Geometry: final body of the model. Coordinates: model frame, mm. A direction names the side the tool comes from. Give positions to 0.01 mm unless a question says otherwise; leave off trailing zeros. Order: outer loops, then holes, each group sorted by start corner. A loop starts at its lowest first (then second) coordinate and runs counter-clockwise, first axis right, second up. Notation, with made-up numbers: (-16, 37.25) - (-1, 37.25) arc R30 ccw to (-1, 70.25) - close; hole circle Ø6 at (38.25, 65). An arc over 180 degrees is marked (long way). Put each result on its own line as item: value. Start each with the question number.
1. Mould query, pull axis Z, two halves, no side actions, for faces 1 (the flat face through (0, -42, 20)), 2 (the flat face through (-5.5, 53, 12)), 3 (the flat face through (10.25, -78, -11)). Classes: pulls with the +Z half, pulls with the -Z half, needs draft (parallel to the pull), parting line crosses it, or undercut.
2. Section D-D on y = 0. Return the cut outline in (x, z), plus the area to 3 significant figures.
3. First-contact query: P1, Ø8.5, axis at x = 7.5, y = 54.5, coming from the -Z side; P2, Ø8, axis at y = 42.5, z = 5, coming from the +X side; P3, Ø9, axis at y = 58, z = 14.5, coming from the +X side; P4, Ø10, axis at x = -32, z = -8, coming from the -Y side. Flat tips, straight axial feed; report the tip coordinate or a pass-through.
4. Set-up query: faces 4 (the flat face through (0, -61.5, -21)), 5 (the flat face through (-17.5, -72, 1)), 6 (the flat face through (17.5, -73, 1)), 7 (the flat face through (7.25, -77, -18)), 8 (the flat face through (5, 49, 0.25)). Return all of +Z, -Z, +X, -X, +Y, -Y with unobstructed straight access to the full face (end or side cutting, diameter ignored); none if empty.
5. Ray query, line 1 along X through (y, z) = (0, 16); line 2 along Y through (x, z) = (-3, 10); line 3 along Z through (x, y) = (6, -62.5). Return the intervals inside material, ascending. Write a range as from..to.
6. Section A-A on z = -18. Return the cut outline in (x, y).
7. Section B-B on x = 0. Return the cut outline in (y, z), plus the area to 3 significant figures.
8. Section C-C on z = 10. Return the cut outline in (x, y).
Autodesk Inventor part; units mm, degrees
ref_plane "YZ Plane" through (0, 0, 0) normal (1, 0, 0) x (0, 1, 0)
ref_plane "XZ Plane" through (0, 0, 0) normal (0, 1, 0) x (-1, 0, 0)
ref_plane "XY Plane" through (0, 0, 0) normal (0, 0, 1) x (1, 0, 0)
sketch "Sketch1" plane through (0, 0, 0) normal (0, 0, 1) x (1, 0, 0)
  arc A0 (-2.5, 41.4246) -> (2.5, 41.4246) centre (0, 0) ccw
  arc A1 (-5.5, 46.1736) -> (5.5, 46.1736) centre (0, 0) ccw
  line L0 (-2.5, 61.4493) -> (2.5, 61.4493)
  line L1 (2.5, 61.4493) -> (2.5, 41.4246)
  line L2 (-2.5, 41.4246) -> (-2.5, 61.4493)
  line L3 (5.5, 46.1736) -> (5.5, 64.4493)
  line L4 (-5.5, 64.4493) -> (-5.5, 46.1736)
  line L5 (-2.5, 61.4493) -> (-2.5, 64.4493)
  line L6 (2.5, 61.4493) -> (2.5, 64.4493)
  line L7 (5.5, 64.4493) -> (2.5, 64.4493)
  line L8 (-2.5, 64.4493) -> (-5.5, 64.4493)
  line L9 (-17.5, -41.5) -> (17.5, -41.5)
  line L10 (17.5, -41.5) -> (17.5, -91.5)
  line L11 (17.5, -91.5) -> (-17.5, -91.5)
  line L12 (-17.5, -91.5) -> (-17.5, -41.5)
  point P0 (0, 61.4493)
  point P1 (0, -91.5)
  point P2 (-17.5, -43.0813)
  point P3 (17.5, -43.0813)
  point P4 (16.5831, -25)
  point P5 (-16.5831, -25)
  point P6 (0, -41.5)
  dimension "d0" = 83
  dimension "d1" = 93
  dimension "d4" = 3
  dimension "d5" = 5
  dimension "d6" = 3
  dimension "d7" = 3
  dimension "d8" = 35
  dimension "d9" = 50
  dimension "d35" = 15.2757
extrude "Extrusion1" add sketch "Sketch1" along normal blind 20 contours A0 L9 L12 A1 L4 L8 L5 L2 | L9 L10 A1 L12 | A0 L1 L6 L7 L3 A1 L10 L9 | A1 L10 L11 L12
sketch "Sketch2" plane through (5.5, 46.1736, 0) normal (1, 0, 0) x (0, 0, -1)
  line L0 (-20, 0) -> (-20, 18.2757)
  line L1 (0, 18.2757) -> (-20, 18.2757)
  point P0 (0, -46.1736)
  point P1 (-10, 9.1378)
  point P2 (-20, 9.1378)
  point P3 (-10, 18.2757)
hole "Hole1" at (5.5, 55.3114, 10) direction (-1, 0, 0) diameter 5 end through all
sketch "Sketch3" plane through (0, 0, 0) normal (0, 0, -1) x (-1, 0, 0)
  arc A0 (-5.5, 46.1736) -> (-17.5, -43.0813) centre (0, 0) ccw
  line L0 (5.5, 64.4493) -> (5.5, 46.1736)
  line L1 (2.5, 64.4493) -> (5.5, 64.4493)
  line L2 (2.5, 41.4246) -> (2.5, 64.4493)
  arc A1 (-2.5, 41.4246) -> (2.5, 41.4246) centre (0, 0) ccw
  line L3 (-2.5, 64.4493) -> (-2.5, 41.4246)
  line L4 (-5.5, 64.4493) -> (-2.5, 64.4493)
  line L5 (-5.5, 46.1736) -> (-5.5, 64.4493)
  arc A2 (-5.5, 46.1736) -> (-17.5, -43.0813) centre (0, 0) ccw
  arc A3 (17.5, -43.0813) -> (5.5, 46.1736) centre (0, 0) ccw
  line L6 (-17.5, -58.6416) -> (17.5, -58.6416)
  arc A4 (17.5, -43.0813) -> (5.5, 46.1736) centre (0, 0) ccw
  line L7 (-17.5, -91.5) -> (-17.5, -43.0813)
  line L8 (17.5, -91.5) -> (-17.5, -91.5)
  line L9 (17.5, -43.0813) -> (17.5, -91.5)
  point P0 (16.5831, -25)
  point P1 (-16.5831, -25)
  point P2 (17.5, -58.6416)
  point P3 (-17.5, -58.6416)
  dimension "d36" = 32.8584
extrude "Extrusion2" add sketch "Sketch3" along normal blind 30 contours L6 L9 L8 L7
sketch "Sketch4" plane through (17.5, -91.5, 20) normal (1, 0, 0) x (0, 0, -1)
  line L0 (50, 32.8584) -> (20, 32.8584)
  line L1 (20, 32.8584) -> (20, 30)
  line L2 (20, 30) -> (50, 30)
  line L3 (50, 30) -> (50, 32.8584)
  line L4 (50, 0) -> (0, 0)
  line L5 (50, 32.8584) -> (50, 0)
  line L6 (20, 32.8584) -> (50, 32.8584)
  line L7 (20, 32.8584) -> (20, 48.4187)
  point P0 (20, 91.5)
  point P1 (20, 0)
  point P2 (20, 60)
  dimension "d22" = 30
extrude "Extrusion3" cut sketch "Sketch4" against normal through all
sketch "Sketch6" plane through (-17.5, -91.5, 20) normal (0, -1, 0) x (1, 0, 0)
  line L0 (27.5, -35) -> (24.5, -35)
  line L1 (24.5, -35) -> (24.5, -40)
  line L2 (24.5, -40) -> (10.5, -40)
  line L3 (10.5, -40) -> (10.5, -35)
  line L4 (10.5, -35) -> (7.5, -35)
  line L5 (7.5, -35) -> (7.5, -20)
  line L6 (7.5, -20) -> (27.5, -20)
  line L7 (27.5, -20) -> (27.5, -35)
  line L8 (27.75, -19.75) -> (7.25, -19.75)
  line L9 (7.25, -19.75) -> (7.25, -35.25)
  line L10 (7.25, -35.25) -> (10.25, -35.25)
  line L11 (10.25, -35.25) -> (10.25, -40.25)
  line L12 (10.25, -40.25) -> (24.75, -40.25)
  line L13 (24.75, -40.25) -> (24.75, -35.25)
  line L14 (24.75, -35.25) -> (27.75, -35.25)
  line L15 (27.75, -35.25) -> (27.75, -19.75)
  point P0 (17.5, -20)
  dimension "d28" = 0.25
extrude "Extrusion5" cut sketch "Sketch6" against normal through all contours L0 L1 L2 L3 L4 L5 L6 L7 | L15 L14 L13 L12 L11 L10 L9 L8
sketch "Sketch9" plane through (10.25, -91.5, -15.25) normal (-1, 0, 0) x (0, 0, 1)
  line L0 (10.25, 30) -> (5.25, 30)
  line L1 (5.25, 30) -> (5.25, 10)
  line L2 (5.25, 10) -> (10.25, 10)
  line L3 (10.25, 10) -> (10.25, 30)
  line L4 (0, 30) -> (15.25, 30)
  line L5 (15.5, 0) -> (0, 0)
  point P0 (15.25, 91.5)
  point P1 (7.75, 10)
  point P2 (7.75, 0)
  point P3 (15.5, 25)
  dimension "d31" = 5
  dimension "d32" = 20
extrude "Extrusion6" cut sketch "Sketch9" against normal through all
chamfer "Chamfer1" distance 2 angle 45 2 edges at (-17.5, -61.5, -15) (17.5, -61.5, -20)
properties part number "0008-10-055 Doking"
Resolved:
1. face 1: pulls with the +Z half
1. face 2: needs draft
1. face 3: undercut
2. outline: (-46.5, 0) - (-41.5, 0) - (-41.5, 20) - (-46.5, 20) - close; (41.5, 0) - (46.5, 0) - (46.5, 20) - (41.5, 20) - close
2. area: 200 mm^2
3. P1: z = 0.25
3. P2: x = 26.08
3. P3: x = 5.5
3. P4: through
4. face 4: -Z, +X, -X, +Y
4. face 5: +Z, -Z, -X, -Y
4. face 6: +Z, -Z, +X, -Y
4. face 7: +Y, -Y
4. face 8: -Z, +Y, -Y
5. line 1: -46.5..-41.5, 41.5..46.5
5. line 2: -91.5..-41.39, 41.39..52.81, 57.81..64.45
5. line 3: -30..-20.25, 0.25..20
6. outline: (-17.5, -91.5) - (-7.25, -91.5) - (-7.25, -61.5) - (-15.5, -61.5) - (-17.5, -63.5) - close; (7.25, -91.5) - (17.5, -91.5) - (17.5, -63.5) - (15.5, -61.5) - (7.25, -61.5) - close
7. outline: (-91.5, -30) - (-61.5, -30) - (-61.5, -20.25) - (-91.5, -20.25) - close; (-91.5, 0.25) - (-41.5, 0.25) - (-41.5, 20) - (-91.5, 20) - close
7. area: 1,280 mm^2
8. outline: (-17.5, -91.5) - (17.5, -91.5) - (17.5, -43.08) arc R46.5 ccw to (5.5, 46.17) - (5.5, 52.81) - (2.5, 52.81) - (2.5, 41.42) arc R41.5 cw (long way) to (-2.5, 41.42) - (-2.5, 52.81) - (-5.5, 52.81) - (-5.5, 46.17) arc R46.5 ccw to (-17.5, -43.08) - close; (-5.5, 57.81) - (-2.5, 57.81) - (-2.5, 64.45) - (-5.5, 64.45) - close; (2.5, 57.81) - (5.5, 57.81) - (5.5, 64.45) - (2.5, 64.45) - close
